Build history of the part. All positions in model axes, mm. A direction names the side the tool comes from. Give positions to 0.01 mm unless a question says otherwise; leave off trailing zeros. Loops run counter-clockwise (first coordinate to the right, second up) from the corner with the lowest first, then second, coordinate; pieces in that order, holes last.
1) Band-saw the part on A-A on z = 22.25. List the corners of the cut face in (x, y), then the cut area to 3 significant figures.
2) Band-saw the part on B-B on y = 3.3. List the corners of the cut face in (x, z).
3) Wall check: line 1 (X direction, y = 0.5, z = 22); line 2 (Z direction, x = 37, y = 0.2); line 3 (Z direction, x = 67.5, y = 0.4). Give the ranges that are in metal, low to high.
4) Flat gauge pins, fed straight in: P1, Ø2, axis at y = 2, z = 23.5, coming from the -X side; P2, Ø1.2, axis at x = 51, y = 2, coming from the +Z side; P3, Ø2, axis at y = 2.5, z = 23.5, coming from the +X side; P4, Ø2, axis at x = 37, y = 2.5, coming from the -Z side. Where does each tip first touch, or does it go through?
5) Two-plate mould, pull along X, no slides. Class faces 6 (the flat face through (36, 2, 0)), 7 (the flat face through (46, 2, -4)), 8 (the flat face through (75, 2, 11)): +X half, -X half, draft (parallel to the pull), parting line (faces both ways), or undercut.
6) 3-axis set-ups, long thin cutter, end or side, ignore diameter. For faces 1 (the flat face through (45, 2, 23)), 2 (the flat face through (71, 2, -2)), 3 (the flat face through (78, 2, 8)), 4 (the flat face through (73, 2, 21)), 5 (the flat face through (41, 2, -2)): which of +Z, -Z, +X, -X, +Y, -Y reach the whole face in a straight line?
7) Band-saw the part on C-C on x = 17. List the corners of the cut face in (y, z), then the cut area to 3 significant figures.
```python
from build123d import *

# Parameters (mm, degrees)
SKETCH1_W           = 75
SKETCH1_H           = 21
BOSS_EXTRUDE1_DEPTH = 4
SKETCH2_W           = 8
SKETCH2_H           = 4
BOSS_EXTRUDE2_DEPTH = 6
SKETCH3_W           = 10
SKETCH3_H           = 4
BOSS_EXTRUDE3_DEPTH = 4
LPATTERN1_COUNT     = 4
LPATTERN1_PITCH     = 20
SKETCH4_W           = 1
SKETCH4_H           = 4
BOSS_EXTRUDE4_DEPTH = 4
SKETCH5_W           = 45
SKETCH5_H           = 4
SKETCH5_W_2         = 10
BOSS_EXTRUDE5_DEPTH = 4


with BuildPart() as part:
    # Sketch1 → Boss-Extrude1 (new body)
    with BuildSketch(Plane(origin=(0, 0, 0), x_dir=(1, 0, 0), z_dir=(0, 1, 0))):
        with Locations((37.5, -10.5)):
            Rectangle(SKETCH1_W, SKETCH1_H)
    extrude(amount=BOSS_EXTRUDE1_DEPTH)

    # Sketch2 → Boss-Extrude2 (add)
    with BuildSketch(Plane(origin=(75, 0, 0), x_dir=(0, 0, -1), z_dir=(1, 0, 0))):
        with Locations((-17, 2)):
            Rectangle(SKETCH2_W, SKETCH2_H)
        with Locations((-4, 2)):
            Rectangle(SKETCH2_W, SKETCH2_H)
    extrude(amount=BOSS_EXTRUDE2_DEPTH)

    # Sketch3 → Boss-Extrude3 (add, through all)
    with BuildSketch(Plane(origin=(0, 4, 0), x_dir=(1, 0, 0), z_dir=(0, 1, 0))):
        with Locations((66, 2)):
            Rectangle(SKETCH3_W, SKETCH3_H)
    boss_extrude3 = extrude(amount=-BOSS_EXTRUDE3_DEPTH)

    # LPattern1: Boss-Extrude3 ×4
    with Locations(*[(-i * LPATTERN1_PITCH, 0, 0) for i in range(1, LPATTERN1_COUNT)]):
        add(boss_extrude3)

    # Sketch4 → Boss-Extrude4 (add, through all)
    with BuildSketch(Plane(origin=(0, 4, 0), x_dir=(1, 0, 0), z_dir=(0, 1, 0))):
        with Locations((0.5, 2)):
            Rectangle(SKETCH4_W, SKETCH4_H)
    extrude(amount=-BOSS_EXTRUDE4_DEPTH)

    # Sketch5 → Boss-Extrude5 (add, through all)
    with BuildSketch(Plane(origin=(0, 4, 0), x_dir=(1, 0, 0), z_dir=(0, 1, 0))):
        with Locations((22.5, -23)):
            Rectangle(SKETCH5_W, SKETCH5_H)
        with Locations((60, -23)):
            Rectangle(SKETCH5_W_2, SKETCH5_H)
    extrude(amount=-BOSS_EXTRUDE5_DEPTH)


solid = part.part
```
Findings below:
1. outline: (0, 0) - (45, 0) - (45, 4) - (0, 4) - close; (55, 0) - (65, 0) - (65, 4) - (55, 4) - close
1. area: 220 mm2
2. outline: (0, -4) - (11, -4) - (11, 0) - (21, 0) - (21, -4) - (31, -4) - (31, 0) - (41, 0) - (41, -4) - (51, -4) - (51, 0) - (61, 0) - (61, -4) - (71, -4) - (71, 0) - (81, 0) - (81, 8) - (75, 8) - (75, 13) - (81, 13) - (81, 21) - (65, 21) - (65, 25) - (55, 25) - (55, 21) - (45, 21) - (45, 25) - (0, 25) - close
3. line 1: x = 0 to 45, 55 to 65
3. line 2: z = 0 to 25
3. line 3: z = -4 to 21
4. P1: stops at x = 0
4. P2: stops at z = 21
4. P3: stops at x = 65
4. P4: stops at z = 0
5. face 6: undercut
5. face 7: draft
5. face 8: +X half
6. face 1: +Z, +Y, -Y
6. face 2: -Z, +X, +Y, -Y
6. face 3: +X, +Y, -Y
6. face 4: +Z, +X, +Y, -Y
6. face 5: -Z, +Y, -Y
7. outline: (0, 0) - (4, 0) - (4, 25) - (0, 25) - close
7. area: 100 mm2
